from build123d import *

# Parameters (mm, degrees)
F0_W      = 60
F0_H      = 77
F1_DEPTH  = 70
F2_T      = -3
F3_W      = 21
F3_H      = 25
F3_H_2    = 29
F3_H_3    = 28.8890717719
F4_DEPTH  = 60.001
F5_R      = 1.75
F6_DEPTH  = 3.001
F3_R      = 3.175
F7_DEPTH  = 60.001
F8_R      = 3.175
F8_W      = 24
F8_H      = 56.7587303836
F9_DEPTH  = 77.001
F10_DEPTH = 77.001


# Not quite as in the source:
# - a feature names something its author has since deleted; it is built from what else it names


with BuildPart() as f1:
    # F0 (on Top) → F1 (new body)
    with BuildSketch(Plane.XY):
        Rectangle(F0_W, F0_H)
    extrude(amount=F1_DEPTH)

    # F2
    f2_openings = [f1.faces().sort_by_distance(p)[0] for p in [
        (0, 0, 70),
    ]]
    offset(amount=F2_T, openings=f2_openings)

    # F3 (on face) → F4 (cut, through all)
    with BuildSketch(Plane.YZ.offset(30)):
        with Locations((-25, 47.5)):
            Rectangle(F3_W, F3_H)
        with Locations((-1, 47.5)):
            Rectangle(F3_W, F3_H)
        with Locations((23, 47.5)):
            Rectangle(F3_W, F3_H)
        with Locations((-25, 17.5)):
            Rectangle(F3_W, F3_H_2)
        with Locations((-1, 17.5554641141)):
            Rectangle(F3_W, F3_H_3)
        with Locations((23, 17.5)):
            Rectangle(F3_W, F3_H_2)
    extrude(amount=-F4_DEPTH, mode=Mode.SUBTRACT)

    # F5 (on face) → F6 (cut, through all)
    with BuildSketch(Plane.XY.offset(3)):
        with Locations((-15, -19.25)):
            Circle(F5_R)
        with Locations((10.4, -19.25)):
            Circle(F5_R)
        with Locations((-15, 19.25)):
            Circle(F5_R)
        with Locations((10.4, 19.25)):
            Circle(F5_R)
    extrude(amount=-F6_DEPTH, mode=Mode.SUBTRACT)

    # F3 (on face) → F7 (cut, through all)
    with BuildSketch(Plane.YZ.offset(30)):
        with Locations((0, 65)):
            Circle(F3_R)
    extrude(amount=-F7_DEPTH, mode=Mode.SUBTRACT)

    # F8 (on face) → F9 (cut, through all)
    with BuildSketch(Plane(origin=(0, 38.5, 0), x_dir=(-1, 0, 0), z_dir=(0, 1, 0))):
        with Locations((0, 65)):
            Circle(F8_R)
        with Locations((-15, 31.3793651918)):
            Rectangle(F8_W, F8_H)
        with Locations((15, 31.3793651918)):
            Rectangle(F8_W, F8_H)
    extrude(amount=-F9_DEPTH, mode=Mode.SUBTRACT)

    # F8 (on face) → F10 (cut, through all)
    with BuildSketch(Plane(origin=(0, 38.5, 0), x_dir=(-1, 0, 0), z_dir=(0, 1, 0))):
        with Locations((0, 65)):
            Circle(F8_R)
        with Locations((-15, 31.3793651918)):
            Rectangle(F8_W, F8_H)
        with Locations((15, 31.3793651918)):
            Rectangle(F8_W, F8_H)
    extrude(amount=-F10_DEPTH, mode=Mode.SUBTRACT)


solid = f1.part
Source: CAD feature listing. Evaluate the final solid. Frame: model axes, mm. A direction names the side the tool comes from. Round coordinates to 2 decimals unless told otherwise and drop trailing zeros. Order: outer loops, then holes, each group sorted by start corner. A loop starts at its lowest first (then second) coordinate and runs counter-clockwise, first axis right, second up. Notation, with made-up numbers: (28, 84.5) - (78, 84.5) arc R8 ccw to (78, 96.5) - close; hole circle Ø8 at (83, 47.25). An arc over 180 degrees is marked (long way). Use a Markdown table: item, result. Add a question column.
1. Section query D-D (x = -15). Return the cut outline in (y, z).
2. Section query A-A (y = -19.25). Return the cut outline in (x, z).
3. Line query: probe 1 along Z at (x, y) = (27.5, 28); probe 2 along Y at (x, z) = (-15, 0.85); probe 3 along Z at (x, y) = (29, 0) (3 decimals). Output: solid intervals per line, ascending.
4. Section query C-C (x = 21). Return the cut outline in (y, z).
5. Mould query, pull axis X, two halves, no side actions, for faces 1 (the flat face through (29, 23, 60)), 2 (the flat face through (30, -0.2, 34.8)), 3 (the flat face through (0, -1, 3)). Classes: +X half, -X half, draft (parallel to the pull), parting line (faces both ways), or undercut.
6. Section query B-B (z = 33). Return the cut outline in (x, y), then the cut area to 3 significant figures.
7. Set-up query: faces 4 (the flat face through (-3, -37, 31)), 5 (the flat face through (-28, 23, 60)), 6 (the flat face through (-27, 12, 46)). Return all of +Z, -Z, +X, -X, +Y, -Y with unobstructed straight access to the full face (end or side cutting, diameter ignored); none if empty.
8. First-contact query: pin 1 (2.5 mm diameter, centred on x = 29, y = 22.5, fed in from -Z); pin 2 (3 mm diameter, centred on x = -10, y = 3, fed in from +Z). Flat tips, straight axial feed; report the tip coordinate or a pass-through.
Derived:
| question | item | result |
|---|---|---|
| 1 | outline | (-38.5, 0) - (-21, 0) - (-21, 3) - (-38.5, 3) - close; (-38.5, 59.76) - (-35.5, 59.76) - (-35.5, 70) - (-38.5, 70) - close; (-17.5, 0) - (17.5, 0) - (17.5, 3) - (-17.5, 3) - close; (21, 0) - (38.5, 0) - (38.5, 3) - (21, 3) - close; (35.5, 59.76) - (38.5, 59.76) - (38.5, 70) - (35.5, 70) - close |
| 2 | outline | (-30, 0) - (-16.75, 0) - (-16.75, 3) - (-30, 3) - close; (-30, 32) - (-27, 32) - (-27, 35) - (-30, 35) - close; (-30, 60) - (-27, 60) - (-27, 70) - (-30, 70) - close; (-13.25, 0) - (8.65, 0) - (8.65, 3) - (-13.25, 3) - close; (12.15, 0) - (30, 0) - (30, 3) - (12.15, 3) - close; (27, 32) - (30, 32) - (30, 35) - (27, 35) - close; (27, 60) - (30, 60) - (30, 70) - (27, 70) - close |
| 3 | probe 1 | 0 to 3, 32 to 35, 60 to 70 |
| 3 | probe 2 | -38.5 to -21, -17.5 to 17.5, 21 to 38.5 |
| 3 | probe 3 | 0 to 3.111, 32 to 35, 60 to 61.825, 68.175 to 70 |
| 4 | outline | (-38.5, 0) - (38.5, 0) - (38.5, 3) - (-38.5, 3) - close; (-38.5, 59.76) - (-35.5, 59.76) - (-35.5, 70) - (-38.5, 70) - close; (35.5, 59.76) - (38.5, 59.76) - (38.5, 70) - (35.5, 70) - close |
| 5 | face 1 | draft |
| 5 | face 2 | +X half |
| 5 | face 3 | undercut |
| 6 | outline | (-30, -38.5) - (-27, -38.5) - (-27, 38.5) - (-30, 38.5) - close; (-3, -38.5) - (3, -38.5) - (3, -35.5) - (-3, -35.5) - close; (-3, 35.5) - (3, 35.5) - (3, 38.5) - (-3, 38.5) - close; (27, -38.5) - (30, -38.5) - (30, 38.5) - (27, 38.5) - close |
| 6 | area | 498 mm2 |
| 7 | face 4 | +Y, -Y |
| 7 | face 5 | +X, -X |
| 7 | face 6 | none |
| 8 | pin 1 | z = 0 |
| 8 | pin 2 | z = 3 |
